Can you work these out from the drawing? Everything is in mm from the part's minimum corner. A direction names the side the tool comes from. Round coordinates to 2 decimals unless told otherwise and drop trailing zeros. Write each loop counter-clockwise with the first axis right and the second up, starting at its lowest first coordinate (ties: lowest second). Pieces come first, ordered by that corner, then holes. Notation, with made-up numbers: (56, 55) -> (69, 55) arc R25 ccw to (69, 91) -> close; hole circle Ø2 at (44, -34). An arc over 180 degrees is marked (long way). Answer as CSV lines item,"result".
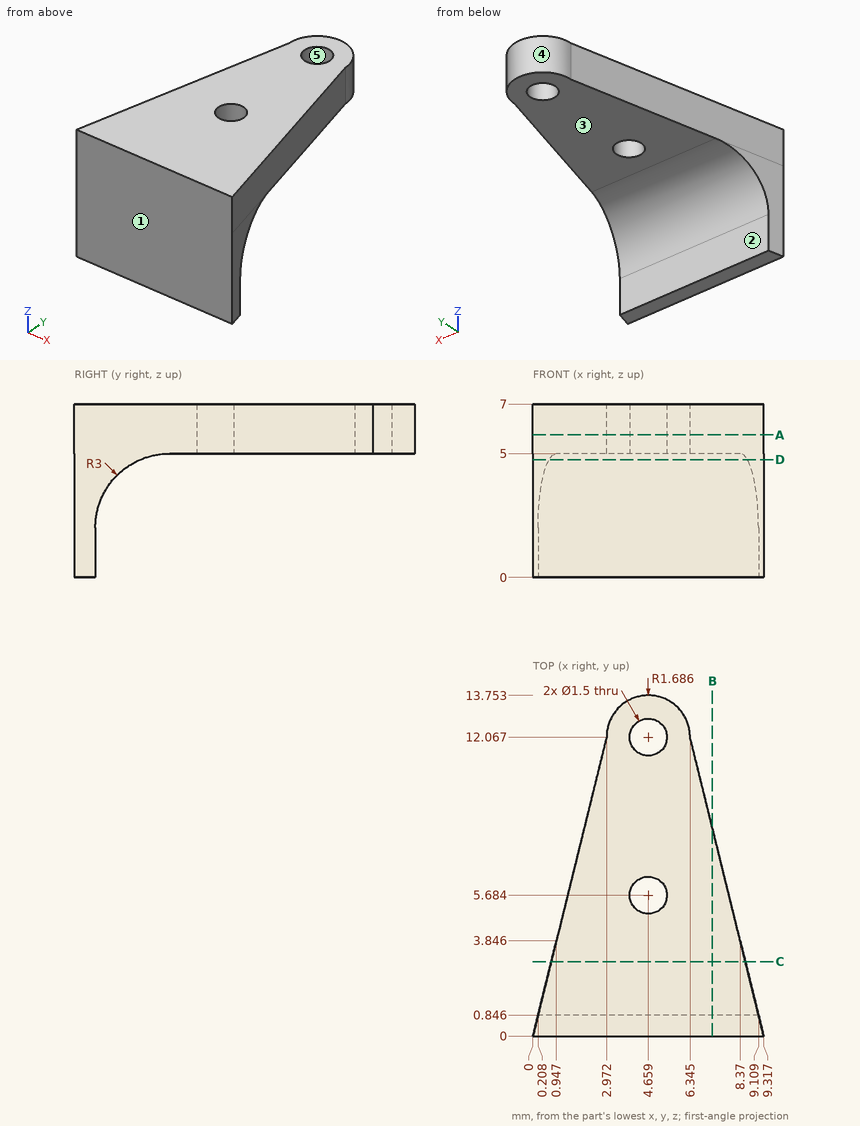
Item 1: For the marked faces 1 and 2, which set-ups out of +Z, -Z, +X, -X, +Y, -Y let a thin tool reach every point of the face, with its end or its side?
Results found:
face 1,"+Z, -Z, +X, -X, -Y"
face 2,"-Z, +X, -X, +Y"
Item 2: I need wall thicknesses on L1, parallel to Y at x = 1, z = 1.25; L2, parallel to Z at x = 2.75, y = 9.25; L3, parallel to Y at x = 7.25, z = 4. Which ranges of each line are inside material? Lowest first, please.
Results found:
L1,"y = 0 to 0.85"
L2,"z = 5 to 7"
L3,"y = 0 to 1.61"
Item 3: Suppose I cut it at C-C, the plane y = 3. List the corners of the cut face in (x, z) for me.
Results found:
outline,"(0.74, 4.88) -> (8.58, 4.88) -> (8.58, 7) -> (0.74, 7) -> close"
Item 4: Suppose I cut it at B-B, the plane x = 7.25. List the corners of the cut face in (y, z) for me.
Results found:
outline,"(0, 0) -> (0.85, 0) -> (0.85, 2) arc R3 cw to (3.85, 5) -> (8.39, 5) -> (8.39, 7) -> (0, 7) -> close"
Item 5: Suppose I cut it at A-A, the plane z = 5.75. State how many separate pieces and enclosed holes the cut face has, then the cut area to 3 significant figures.
Results found:
separate pieces,"1"
enclosed holes,"2"
area,"77.5 mm²"
Item 6: If we mould it in two halves opening along X, with no side actions, what happens to the marked faces 3, 4 and 5? For each: pulls with the +X half, pulls with the -X half, needs draft (parallel to the pull), parting line crosses it, or undercut.
Results found:
face 3,"needs draft"
face 4,"parting line crosses it"
face 5,"undercut"
Item 7: Will these pins go through, and if not, where does the flat tip stop? pin 1 (1.2 mm diameter, centred on x = 4.66, y = 5.68, fed in from +Z); pin 2 (2 mm diameter, centred on x = 5, z = 1.5, fed in from +Y); pin 3 (3.5 mm diameter, centred on x = 4, y = 9, fed in from -Z).
Results found:
pin 1,"passes through"
pin 2,"stops at y = 0.89"
pin 3,"stops at z = 5"
Item 8: Suppose I cut it at D-D, the plane z = 4.75. List the corners of the cut face in (x, y) for me (1 decimal).
Results found:
outline,"(0, 0) -> (9.3, 0) -> (8.7, 2.6) -> (0.7, 2.6) -> close"
